from build123d import *

# Parameters (mm, degrees)
CROQUIS1_R               = 2
CROQUIS1_R_2             = 1.5
CROQUIS1_W               = 75
CROQUIS1_H               = 50
SALIENTE_EXTRUIR4_DEPTH  = 5
CROQUIS3_W               = 5
CROQUIS3_H               = 5
SALIENTE_EXTRUIR5_DEPTH  = 50
CROQUIS4_W               = 3
CROQUIS4_H               = 50
SALIENTE_EXTRUIR7_DEPTH  = 22
SALIENTE_EXTRUIR9_DEPTH  = 27.5
CROQUIS7_W               = 10
CROQUIS7_H               = 5
SALIENTE_EXTRUIR10_DEPTH = 10
CROQUIS8_W               = 10
CROQUIS8_H               = 5
SALIENTE_EXTRUIR11_DEPTH = 10
SALIENTE_EXTRUIR12_DEPTH = 30
CROQUIS10_R              = 0.5
CORTAR_EXTRUIR2_DEPTH    = 43


with BuildPart() as part:
    # Croquis1 → Saliente-Extruir4 (new body)
    # profile 1 of 2: a face of its own
    with BuildSketch(Plane.XY):
        Polygon((-71.5, -27.5), (-71.5, -32.5), (-3.5, -32.5), (-3.5, -27.5), (1.5, -27.5), (1.5, -25), (1.5, 25), (1.5, 27.5), (-3.5, 27.5), (-3.5, 32.5), (-71.5, 32.5), (-71.5, 27.5), (-76.5, 27.5), (-76.5, -27.5), align=None)
        with Locations((-66.5, -22.5)):
            Circle(CROQUIS1_R, mode=Mode.SUBTRACT)
        with Locations((-2, 0)):
            Circle(CROQUIS1_R_2, mode=Mode.SUBTRACT)
        with Locations((-66.5, 22.5)):
            Circle(CROQUIS1_R, mode=Mode.SUBTRACT)
    # profile 2 of 2: a face of its own
    with BuildSketch(Plane.XY):
        with Locations((39, 0)):
            Rectangle(CROQUIS1_W, CROQUIS1_H)
    extrude(amount=SALIENTE_EXTRUIR4_DEPTH)

    # Croquis3 → Saliente-Extruir5 (add)
    with BuildSketch(Plane(origin=(0, 0, 0), x_dir=(-1, 0, 0), z_dir=(0, 0, -1))):
        with Locations((74, 30)):
            Rectangle(CROQUIS3_W, CROQUIS3_H)
        with Locations((1, -30)):
            Rectangle(CROQUIS3_W, CROQUIS3_H)
        with Locations((1, 30)):
            Rectangle(CROQUIS3_W, CROQUIS3_H)
        with Locations((74, -30)):
            Rectangle(CROQUIS3_W, CROQUIS3_H)
    extrude(amount=-SALIENTE_EXTRUIR5_DEPTH)

    # Croquis4 → Saliente-Extruir7 (add)
    with BuildSketch(Plane.XY.offset(5)):
        with Locations((56, 0)):
            Rectangle(CROQUIS4_W, CROQUIS4_H)
    extrude(amount=SALIENTE_EXTRUIR7_DEPTH)

    # Croquis6 → Saliente-Extruir9 (add)
    with BuildSketch(Plane(origin=(0, 0, 0), x_dir=(-1, 0, 0), z_dir=(0, 0, -1))):
        Polygon((-31.5, 13.5), (-31.5, 14.5), (-41.5, 14.5), (-41.5, 13.5), (-41.5, 9.5), (-31.5, 9.5), align=None)
        Polygon((-31.5, -13.5), (-31.5, -9.5), (-41.5, -9.5), (-41.5, -13.5), (-41.5, -14.5), (-31.5, -14.5), align=None)
    extrude(amount=SALIENTE_EXTRUIR9_DEPTH)

    # Croquis7 → Saliente-Extruir10 (add)
    with BuildSketch(Plane(origin=(0, 14.5, 0), x_dir=(1, 0, 0), z_dir=(0, 1, 0))):
        with Locations((36.5, 25)):
            Rectangle(CROQUIS7_W, CROQUIS7_H)
    extrude(amount=SALIENTE_EXTRUIR10_DEPTH)

    # Croquis8 → Saliente-Extruir11 (add)
    with BuildSketch(Plane.XZ.offset(14.5)):
        with Locations((36.5, -25)):
            Rectangle(CROQUIS8_W, CROQUIS8_H)
    extrude(amount=SALIENTE_EXTRUIR11_DEPTH)

    # Croquis9 → Saliente-Extruir12 (add)
    with BuildSketch(Plane(origin=(0, 0, 0), x_dir=(-1, 0, 0), z_dir=(0, 0, -1))):
        with BuildLine():
            Line((69.854101966, -19.5), (76.5, -19.5))
            Line((76.5, -19.5), (76.5, -26.5))
            Line((76.5, -26.5), (68.561552813, -26.5))
            ThreePointArc((68.561552813, -26.5), (70.925192558, -23.317111271), (69.854101966, -19.5))
        make_face()
        with BuildLine():
            Line((68.561552813, 26.5), (76.5, 26.5))
            Line((76.5, 26.5), (76.5, 19.5))
            Line((76.5, 19.5), (69.854101966, 19.5))
            ThreePointArc((69.854101966, 19.5), (70.925192558, 23.317111271), (68.561552813, 26.5))
        make_face()
    extrude(amount=SALIENTE_EXTRUIR12_DEPTH)

    # Croquis10 → Cortar-Extruir2 (cut)
    with BuildSketch(Plane.XZ.offset(14.5)):
        with Locations(Location((37, -4, 0), (0, 0, 270))):
            Circle(CROQUIS10_R)
        with Locations(Location((37, -20, 0), (0, 0, 270))):
            Circle(CROQUIS10_R)
    extrude(amount=-CORTAR_EXTRUIR2_DEPTH, mode=Mode.SUBTRACT)


solid = part.part
Verification items for the finished model (mm, model axes). A direction names the side the tool comes from. Coordinates: 2 decimals unless noted, no trailing zeros. Loops run counter-clockwise (first coordinate to the right, second up) from the corner with the lowest first, then second, coordinate; pieces in that order, holes last. Notation, with made-up numbers: M 75,-3 L 91,-3 A14 cw 91,23 Z; hole C 42,76 d7. An arc over 180 degrees is marked long. One line per item, written item: value.
1. Section check D-D on y = 0. Record the cut outline in (x, z), plus the area to 3 significant figures.
Answers follow:
outline: M -76.5,0 L -3.5,0 L -3.5,5 L -76.5,5 Z; M -0.5,0 L 76.5,0 L 76.5,5 L 57.5,5 L 57.5,27 L 54.5,27 L 54.5,5 L -0.5,5 Z
area: 816 mm^2
2. Set-up check for faces 1 (the flat face through (67, 0, 5)), 2 (the flat face through (-71.5, 30, 27)), 3 (the flat face through (-1, -27.5, 27)), 4 (the flat face through (36, -9.5, -14)), 5 (the flat face through (36, 17, -27.5)): record each of +Z, -Z, +X, -X, +Y, -Y from which the full face is reachable in a straight line by a thin tool's end or side.
Answers follow:
face 1: +Z, +X, +Y, -Y
face 2: +Z, +Y, -Y
face 3: +Z, +X, -X
face 4: -Z, +X, -X
face 5: -Z, +X, +Y, -Y
3. Section check A-A on y = 22.5. Record the cut outline in (x, z).
Answers follow:
outline: M -76.5,-30 L -71,-30 L -71,0 L -68.5,0 L -68.5,5 L -76.5,5 Z; M -64.5,0 L 76.5,0 L 76.5,5 L 57.5,5 L 57.5,27 L 54.5,27 L 54.5,5 L -64.5,5 Z; M 31.5,-27.5 L 41.5,-27.5 L 41.5,-22.5 L 31.5,-22.5 Z
4. Section check C-C on x = -2. Record the cut outline in (y, z), plus the area to 3 significant figures.
Answers follow:
outline: M -32.5,0 L -1.5,0 L -1.5,5 L -27.5,5 L -27.5,50 L -32.5,50 Z; M 1.5,0 L 32.5,0 L 32.5,50 L 27.5,50 L 27.5,5 L 1.5,5 Z
area: 760 mm^2
5. Material ranges on line 1 along Z through (x, y) = (37, -11); line 2 along X through (y, z) = (13, -20); line 3 along Y through (x, z) = (-66, 1), recorded low to high. Write a range as from..to.
Answers follow:
line 1: -27.5..-20.5, -19.5..-4.5, -3.5..5
line 2: 31.5..36.5, 37.5..41.5
line 3: -32.5..-24.44, -20.56..20.56, 24.44..32.5
6. Section check B-B on z = 23. Record the cut outline in (x, y).
Answers follow:
outline: M -76.5,-32.5 L -71.5,-32.5 L -71.5,-27.5 L -76.5,-27.5 Z; M -76.5,27.5 L -71.5,27.5 L -71.5,32.5 L -76.5,32.5 Z; M -3.5,-32.5 L 1.5,-32.5 L 1.5,-27.5 L -3.5,-27.5 Z; M -3.5,27.5 L 1.5,27.5 L 1.5,32.5 L -3.5,32.5 Z; M 54.5,-25 L 57.5,-25 L 57.5,25 L 54.5,25 Z
7. Gauge pin test, flat ends, axial feed: P1, Ø8, axis at x = 36, z = -19, coming from the -Y side; P2, Ø2.5, axis at y = 30.5, z = 26, coming from the +X side; P3, Ø2.5, axis at x = 55.5, y = 9, coming from the +Z side. Record the tip position at first contact, or that the pin passes through.
Answers follow:
P1: y = -24.5
P2: x = 1.5
P3: z = 27
8. Mould release check, pull along Y, two halves, no side actions. Record for faces 6 (the flat face through (76.5, 0, 2)), 7 (the flat face through (-74, -27.5, 27)): pulls with the +Y half, pulls with the -Y half, needs draft (parallel to the pull), parting line crosses it, or undercut.
Answers follow:
face 6: needs draft
face 7: undercut
